Work out the finished part from the listing and answer in its coordinate system (mm). A direction names the side the tool comes from. Give positions to 0.01 mm unless a question says otherwise; leave off trailing zeros. Loops run counter-clockwise (first coordinate to the right, second up) from the corner with the lowest first, then second, coordinate; pieces in that order, holes last. Notation, with made-up numbers: (58.5, 3) -> (107.5, 3) arc R7 cw to (107.5, 15) -> close; hole circle Ø4 at (15.25, 60). An arc over 180 degrees is marked (long way). Answer as CSV lines item,"result". Start each with the question number.
1. Find the intervals of material crossed by line 1 along Z through (x, y) = (-1.75, -3.25); line 2 along Y through (x, z) = (1.75, 3); line 3 along Y through (x, z) = (3, 6), in increasing order.
2. Find section A-A, the plane x = 0. Give the vertices of the cut face in (y, z) (3 decimals).
3. Find section C-C, the plane z = 13. Give the vertices of the cut face in (x, y) (3 decimals), and give its area (3 significant figures).
4. A tool of negligible diameter and unlimited length cuts with its end or side. For faces 1 (the face through (0, 0, 20.4)), 2 (the face through (-2, -3, 4.4)), from which of +Z, -Z, +X, -X, +Y, -Y can it reach the whole face along a straight path? Write none if from no direction.
5. Flat-ended cylindrical pins translate along their axes: pin 1 Ø3 at (y, z) = (4, 15) entering from +X; pin 2 Ø2 at (x, y) = (5, -3.5) entering from -Z; pin 3 Ø5 at (x, z) = (-5, 7.5) entering from -Y. Find the tip coordinate at first contact, or state that the pin passes through.
Autodesk Inventor part; units mm, degrees
ref_plane "YZ Plane" through (0, 0, 0) normal (1, 0, 0) x (0, 1, 0)
ref_plane "XZ Plane" through (0, 0, 0) normal (0, 1, 0) x (-1, 0, 0)
ref_plane "XY Plane" through (0, 0, 0) normal (0, 0, 1) x (1, 0, 0)
sketch "Boceto1" plane through (0, 0, 0) normal (0, 0, 1) x (1, 0, 0)
  circle A0 centre (0, 0) radius 7
  dimension "d0" = 14
extrude "Extrusión1" add sketch "Boceto1" along normal blind 4.4
fillet "Empalme1" radius 2 1 edges at (-7, 0, 0)
sketch "Boceto2" plane through (0, 0, 4.4) normal (0, 0, 1) x (1, 0, 0)
  circle A0 centre (0, 0) radius 3.375
  dimension "d5" = 6.75
extrude "Extrusión2" add sketch "Boceto2" along normal blind 16
properties part number "Socket" material "Aluminio 6061"
Resolved:
1,line 1,"z = 0 to 4.4"
1,line 2,"y = -6.78 to 6.78"
1,line 3,"y = -1.55 to 1.55"
2,outline,"(-7, 2) arc R2 ccw to (-5, 0) -> (5, 0) arc R2 ccw to (7, 2) -> (7, 4.4) -> (3.375, 4.4) -> (3.375, 20.4) -> (-3.375, 20.4) -> (-3.375, 4.4) -> (-7, 4.4) -> close"
3,outline,"circle Ø6.75 at (0, 0)"
3,area,"35.8 mm^2"
4,face 1,"+Z, +X, -X, +Y, -Y"
4,face 2,"+Z"
5,pin 1,"stops at x = 2.27"
5,pin 2,"stops at z = 0"
5,pin 3,"stops at y = -2.27"
